Check sheet for the modelled part. Datum: model origin and axes. Units: mm. Face numbers are marked on the shaded views. A direction names the side the tool comes from. Round coordinates to 2 decimals unless told otherwise and drop trailing zeros. Loops run counter-clockwise (first coordinate to the right, second up) from the corner with the lowest first, then second, coordinate; pieces in that order, holes last. Notation, with made-up numbers: (73.5, -11) - (78.5, -11) arc R36 cw to (78.5, 25) - close; hole circle Ø6 at (-1.75, 7). An arc over 180 degrees is marked (long way). Answer in a Markdown table with one row per item. Add a question column.
(1) Access from +Z, -Z, +X, -X, +Y, -Y to the whole of each face (thin tool, end or side, straight path). Record for the marked faces 1, 2 and 3.
(2) Cross-section at C-C on y = 17. Enter the section's corners in (x, z).
(3) Thickness scan on line 1 along Y through (x, z) = (-2.5, 26.5); line 2 along Y through (x, z) = (12, -41.5); line 3 along Z through (x, y) = (-15, -12.5). Record the ranges inside material, lowest first.
(4) Cross-section at D-D on x = -51. Enter the section's corners in (y, z).
(5) Cross-section at B-B on z = -21. Enter the section's corners in (x, y).
(6) Cross-section at A-A on x = 30. Enter the section's corners in (y, z), then the cut area to 3 significant figures.
(7) Gauge pin test, flat ends, axial feed: pin 1 (10 mm diameter, centred on y = 28, z = -23, fed in from +X); pin 2 (6 mm diameter, centred on x = 36, y = 7, fed in from +Z); pin 3 (1 mm diameter, centred on x = 19, y = 39.5, fed in from -Z). Record the tip position at first contact, or that the pin passes through.
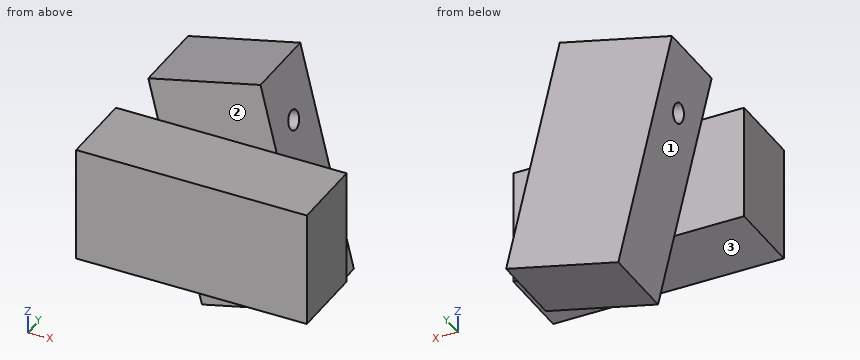
from build123d import *

# Parameters (mm, degrees)
SKETCH1_W           = 120
SKETCH1_H           = 40
BOSS_EXTRUDE1_DEPTH = 30
BOSS_EXTRUDE2_DEPTH = 40
SKETCH3_R           = 5
CUT_EXTRUDE1_DEPTH  = 104.536516906


with BuildPart() as part:
    # Sketch1 → Boss-Extrude1 (new body, symmetric)
    with BuildSketch(Plane.XY):
        Rectangle(SKETCH1_W, SKETCH1_H)
    extrude(amount=BOSS_EXTRUDE1_DEPTH, both=True)

    # Sketch2 → Boss-Extrude2 (add)
    with BuildSketch(Plane(origin=(0, 20, 0), x_dir=(1, 0, 0), z_dir=(0, 1, 0))):
        Polygon((-15.23855654, 65.328297043), (-43.119503711, -51.387823458), (15.23855654, -65.328297043), (43.119503711, 51.387823458), align=None)
    extrude(amount=BOSS_EXTRUDE2_DEPTH)

    # Sketch3 → Cut-Extrude1 (cut, through all)
    with BuildSketch(Plane(origin=(29.179030125, 50, 6.970236793), x_dir=(0.053982445, -0.972634338, -0.225983055), z_dir=(0.972634338, 0, 0.232341226))):
        with Locations((2.700680063, -31.734470672)):
            Circle(SKETCH3_R)
    extrude(amount=-CUT_EXTRUDE1_DEPTH, mode=Mode.SUBTRACT)


solid = part.part
Answers:
| question | item | result |
|---|---|---|
| 1 | face 1 | -Z, -X, +Y |
| 1 | face 2 | +Z, +X, -X, -Y |
| 1 | face 3 | -Z, +X, -X, -Y |
| 2 | outline | (-60, -30) - (60, -30) - (60, 30) - (-60, 30) - close |
| 3 | line 1 | y = -20 to 36.85, 43.15 to 60 |
| 3 | line 2 | y = 20 to 60 |
| 3 | line 3 | z = -30 to 30 |
| 4 | outline | (-20, -30) - (20, -30) - (20, 30) - (-20, 30) - close |
| 5 | outline | (-60, -20) - (60, -20) - (60, 20) - (35.86, 20) - (35.86, 60) - (-25.83, 60) - (-25.83, 20) - (-60, 20) - close |
| 6 | outline | (-20, -30) - (20, -30) - (20, -54.52) - (60, -54.52) - (60, 3.53) - (20, 3.53) - (20, 30) - (-20, 30) - close |
| 6 | area | 4,720 mm^2 |
| 7 | pin 1 | stops at x = 37.53 |
| 7 | pin 2 | stops at z = 30 |
| 7 | pin 3 | stops at z = -57.27 |
